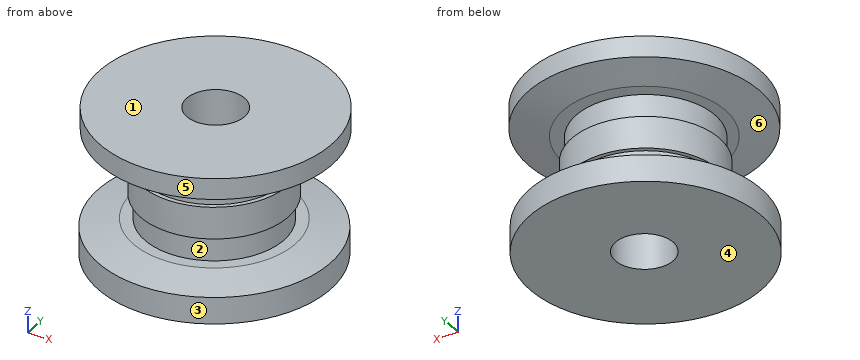
from build123d import *

# Parameters (mm, degrees)
F0_R      = 20
F1_DEPTH  = 6
F2_R      = 12
F3_DEPTH  = 4.25
F4_R      = 12.75
F5_DEPTH  = 5.5
F6_R      = 12
F8_DEPTH  = 4.25
F10_R     = 20
F11_DEPTH = 5
F12_R     = 5
F13_DEPTH = 25.001
F14_SIZE2 = 1.4
F14_SIZE  = 6
F15_SIZE2 = 6
F15_SIZE  = 1.4


with BuildPart() as f1:
    # F0 (on Top) → F1 (new body)
    with BuildSketch(Plane.XY):
        with Locations((-4.7043012455, 29.0725808591)):
            Circle(F0_R)
    extrude(amount=F1_DEPTH)

    # F2 (on face) → F3 (join)
    with BuildSketch(Plane.XY.offset(6)):
        with Locations((-4.7043012455, 29.0725808591)):
            Circle(F2_R)
    extrude(amount=F3_DEPTH)

    # F4 (on face) → F5 (join)
    with BuildSketch(Plane.XY.offset(10.25)):
        with Locations((-4.7043012455, 29.0725808591)):
            Circle(F4_R)
    extrude(amount=F5_DEPTH)

    # F6 (on face) → F8 (join)
    with BuildSketch(Plane.XY.offset(15.75)):
        with Locations((-4.7043012455, 29.0725808591)):
            Circle(F6_R)
    extrude(amount=F8_DEPTH)

    # F10 (on face) → F11 (join)
    with BuildSketch(Plane.XY.offset(20)):
        with Locations((-4.7043012455, 29.4489245862)):
            Circle(F10_R)
    extrude(amount=F11_DEPTH)

    # F12 (on face) → F13 (cut, through all)
    with BuildSketch(Plane.XY.offset(25)):
        with Locations((-4.7043012455, 29.4489245862)):
            Circle(F12_R)
    extrude(amount=-F13_DEPTH, mode=Mode.SUBTRACT)

    # F14
    f14_edges = [f1.edges().sort_by_distance(p)[0] for p in [
        (-24.704301, 29.072581, 6),
    ]]
    f14_side = f1.faces().sort_by_distance((-24.138616, 29.072581, 6))[0]
    chamfer(f14_edges, length=F14_SIZE, length2=F14_SIZE2, reference=f14_side)

    # F15
    f15_edges = [f1.edges().sort_by_distance(p)[0] for p in [
        (-24.704301, 29.448925, 20),
    ]]
    f15_side = f1.faces().sort_by_distance((-24.704301, 29.448925, 22.5))[0]
    chamfer(f15_edges, length=F15_SIZE, length2=F15_SIZE2, reference=f15_side)


solid = f1.part
Geometry check sheet. Reference: the model listing, model coordinates, mm. Face numbers are marked on the shaded views. A direction names the side the tool comes from. Give positions to 0.01 mm unless a question says otherwise; leave off trailing zeros. Write each loop counter-clockwise with the first axis right and the second up, starting at its lowest first coordinate (ties: lowest second). Pieces come first, ordered by that corner, then holes. Notation, with made-up numbers: (-22, 84.25) - (32, 84.25) arc R33 cw to (32, 119.25) - close; hole circle Ø7 at (71.5, 28.25). An arc over 180 degrees is marked (long way). Put each result on its own line as item: value.
1. Sectioned sample at B-B, the plane z = 22.25. Enter the section's corners in (x, y).
Ans:
outline: circle Ø40 at (-4.7, 29.45); hole circle Ø10 at (-4.7, 29.45)
2. Go/stop test with flat-tipped pins: pin 1 (2 mm diameter, centred on x = -9.5, z = 14.5, fed in from +Y); pin 2 (4 mm diameter, centred on x = 9, z = 15.5, fed in from +Y); pin 3 (6 mm diameter, centred on y = 33, z = 10, fed in from -X). Record where each tip stops, or that it passes through.
Ans:
pin 1: stops at y = 41.24
pin 2: stops at y = 34.13
pin 3: stops at x = -17.42
3. Draft check along Z on the marked faces 1, 2 and 3. Enter one of: +Z half, -Z half, draft (parallel to the pull), parting line (faces both ways), or undercut.
Ans:
face 1: +Z half
face 2: undercut
face 3: draft
4. Set-up check for the marked faces 4, 5 and 6: record each of +Z, -Z, +X, -X, +Y, -Y from which the full face is reachable in a straight line by a thin tool's end or side.
Ans:
face 4: -Z, +X, -X, +Y, -Y
face 5: +Z
face 6: none
5. Thickness scan on line 1 (Y direction, x = -4.5, z = 19.5); line 2 (Z direction, x = 5.5, y = 38.5); line 3 (Z direction, x = -5.5, y = 48). Record the ranges inside material, lowest first.
Ans:
line 1: y = 17.07 to 24.45, 34.44 to 41.07
line 2: z = 0 to 6, 20 to 25
line 3: z = 0 to 4.85, 21.07 to 25
6. Sectioned sample at A-A, the plane z = 15.25. Enter the section's corners in (x, y).
Ans:
outline: circle Ø25.5 at (-4.7, 29.07); hole circle Ø10 at (-4.7, 29.45)
